Verification items for this drawing (mm, ordinates from the low corner). A direction names the side the tool comes from. Coordinates: 2 decimals unless noted, no trailing zeros. Write each loop counter-clockwise with the first axis right and the second up, starting at its lowest first coordinate (ties: lowest second). Pieces come first, ordered by that corner, then holes. Notation, with made-up numbers: (39.5, 19) -> (94.5, 19) arc R21 ccw to (94.5, 41) -> close; hole circle Ø6 at (-27.75, -13.75). An arc over 180 degrees is marked (long way). One line per question, with ' | ' between items.
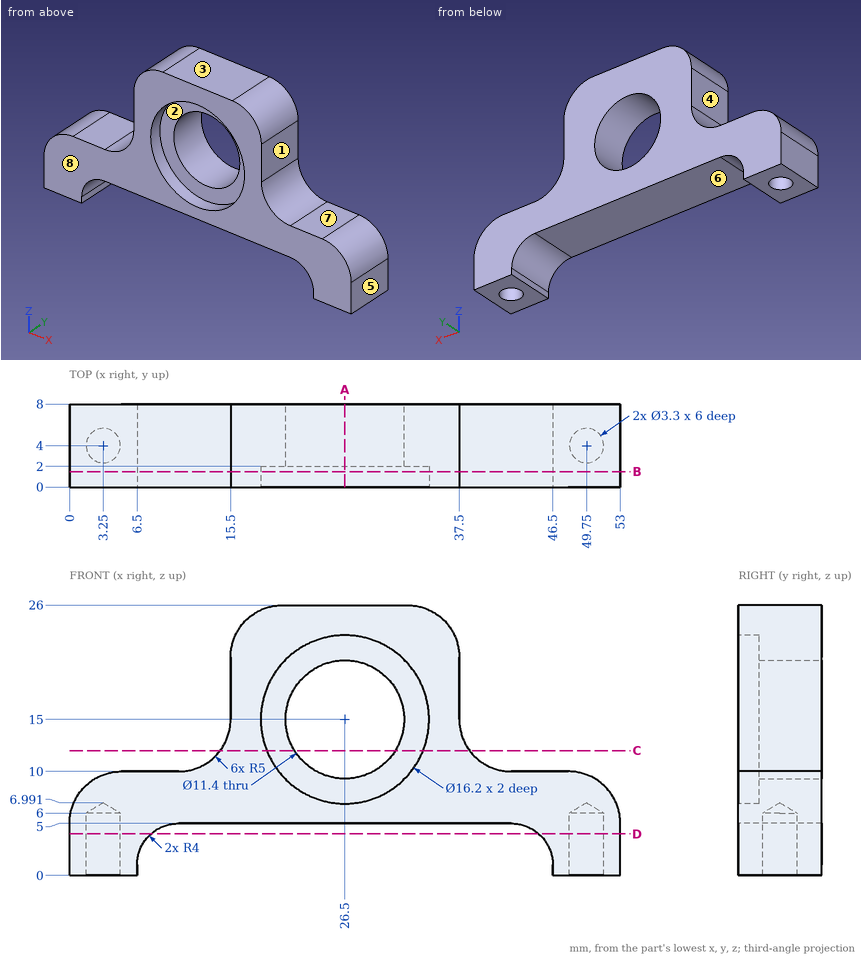
(1) Tool access check on the marked faces 4, 5, 6, 7 and 8. Record the directions out of +Z, -Z, +X, -X, +Y, -Y that give a thin tool (end or side, any length) a straight path to the whole face; none if there is none.
Answers below:
face 4: +Z, -X, +Y, -Y | face 5: +Z, -Z, +X, +Y, -Y | face 6: -Z, +Y, -Y | face 7: +Z, +X, +Y, -Y | face 8: +Z, -Z, +X, -X, -Y
(2) Cross-section at A-A (x = 26.5). Record the cut outline in (y, z), plus the area to 3 significant figures.
Answers below:
outline: (0, 5) -> (8, 5) -> (8, 9.3) -> (2, 9.3) -> (2, 6.9) -> (0, 6.9) -> close; (0, 23.1) -> (2, 23.1) -> (2, 20.7) -> (8, 20.7) -> (8, 26) -> (0, 26) -> close | area: 67.2 mm²
(3) Depth check by flat-ended pin: P1, Ø2, axis at x = 49.75, y = 4, coming from the -Z side; P2, Ø1.6, axis at x = 6.5, y = 4, coming from the +Z side; P3, Ø12, axis at x = 38, z = 11.5, coming from the -Y side; P4, Ø1.5, axis at y = 2, z = 23.5, coming from the -X side. Enter the tip coordinate at first touch or a pass-through.
Answers below:
P1: stops at z = 6.39 | P2: stops at z = 10 | P3: stops at y = 0 | P4: stops at x = 15.82
(4) Cross-section at D-D (z = 4). Count the separate pieces of the cut face and the enclosed holes in it.
Answers below:
separate pieces: 2 | enclosed holes: 2
(5) Cross-section at C-C (z = 12). Record the cut outline in (x, y), plus the area to 3 significant figures.
Answers below:
outline: (14.5, 0) -> (18.98, 0) -> (18.98, 2) -> (21.65, 2) -> (21.65, 8) -> (14.5, 8) -> close; (31.35, 2) -> (34.02, 2) -> (34.02, 0) -> (38.5, 0) -> (38.5, 8) -> (31.35, 8) -> close | area: 104 mm²
(6) Cross-section at B-B (y = 1.5). Record the cut outline in (x, z), plus the area to 3 significant figures.
Answers below:
outline: (0, 0) -> (6.5, 0) -> (6.5, 1) arc R4 cw to (10.5, 5) -> (42.5, 5) arc R4 cw to (46.5, 1) -> (46.5, 0) -> (53, 0) -> (53, 5) arc R5 ccw to (48, 10) -> (42.5, 10) arc R5 cw to (37.5, 15) -> (37.5, 21) arc R5 ccw to (32.5, 26) -> (20.5, 26) arc R5 ccw to (15.5, 21) -> (15.5, 15) arc R5 cw to (10.5, 10) -> (5, 10) arc R5 ccw to (0, 5) -> close; hole circle Ø16.2 at (26.5, 15) | area: 472 mm²
(7) Material ranges on line 1 (X direction, y = 4, z = 1.3); line 2 (Y direction, x = 3.25, z = 4.85); line 3 (Z direction, x = 26.5, y = 4), recorded low to high.
Answers below:
line 1: x = 0 to 1.6, 4.9 to 6.51, 46.49 to 48.1, 51.4 to 53 | line 2: y = 0 to 2.35, 5.65 to 8 | line 3: z = 5 to 9.3, 20.7 to 26
(8) Draft check along Z on the marked faces 1, 2 and 3. Enter one of: pulls with the +Z half, pulls with the -Z half, needs draft (parallel to the pull), parting line crosses it, or undercut.
Answers below:
face 1: needs draft | face 2: undercut | face 3: pulls with the +Z half
